Read the model definition and answer for the solid it produces. Units are mm, in the model's axes. A direction names the side the tool comes from. Coordinates: 2 decimals unless noted, no trailing zeros. Loops run counter-clockwise (first coordinate to the right, second up) from the corner with the lowest first, then second, coordinate; pieces in that order, holes last. Notation, with made-up numbers: M -30,-30 L -6,-30 A16 ccw -6,-6 Z; hole C 56,-19 d9. An arc over 180 degrees is marked long. Put each result on its own line as item: value.
from build123d import *

# Parameters (mm, degrees)
BOX_EXTRUDE_DEPTH             = 100
BOX_EXTRUDE_DEPTH_BACK        = 15
SKETCH2_W                     = 160
SKETCH2_H                     = 140
BOX_INNER_CUT_START           = -20
SKETCH3_W                     = 120
SKETCH3_H                     = 100
BOX_INNER_CUT_DEPTH           = 40
SHAFT_CUT_START               = -60
SKETCH6_R                     = 6
SHAFT_CUT_DEPTH               = 40
BEARING_CUTS_INSIDE_BOX_START = -60
SKETCH9_R                     = 8
SKETCH9_R_2                   = 16
BEARING_CUTS_INSIDE_BOX_DEPTH = 10
SKETCH11_W                    = 120
SKETCH11_H                    = 10
SCISSOR_CUT_DEPTH             = 20
SKETCH12_R                    = 16
MOTOR_HOLE_CUT_DEPTH          = 3.15
RIGHT_SHAFT_LID_CUT_REACH     = 156.306
SKETCH15_R                    = 6
LEFT_BEARING_LID_CUT_START    = -10
SKETCH18_R                    = 8
LEFT_BEARING_LID_CUT_DEPTH    = 10
OUTER_EDGES_FILLET_R          = 4


with BuildPart() as part:
    # Sketch2 → BOX_EXTRUDE (new, two sides: drawn at the far end of the back side and taken through both)
    with BuildSketch(Plane(origin=(0, 0, 0), x_dir=(1, 0, 0), z_dir=(0, 1, 0)).offset(-BOX_EXTRUDE_DEPTH_BACK)):
        Rectangle(SKETCH2_W, SKETCH2_H)
    extrude(amount=BOX_EXTRUDE_DEPTH + BOX_EXTRUDE_DEPTH_BACK)

    # Sketch3 → BOX_INNER_CUT (cut)
    with BuildSketch(Plane(origin=(0, 100, 0), x_dir=(1, 0, 0), z_dir=(0, 1, 0)).offset(BOX_INNER_CUT_START)):
        Rectangle(SKETCH3_W, SKETCH3_H)
    extrude(amount=-BOX_INNER_CUT_DEPTH, mode=Mode.SUBTRACT)

    # Sketch6 → SHAFT_CUT (cut)
    with BuildSketch(Plane(origin=(0, 100, 0), x_dir=(1, 0, 0), z_dir=(0, 1, 0)).offset(SHAFT_CUT_START)):
        with Locations(Location((15, 0, 0), (0, 0, 270))):
            Circle(SKETCH6_R)
        with Locations(Location((-15, 0, 0), (0, 0, 90))):
            Circle(SKETCH6_R)
    extrude(amount=-SHAFT_CUT_DEPTH, mode=Mode.SUBTRACT)

    # Sketch9 → BEARING_CUTS_INSIDE_BOX (cut)
    with BuildSketch(Plane(origin=(0, 100, 0), x_dir=(1, 0, 0), z_dir=(0, 1, 0)).offset(BEARING_CUTS_INSIDE_BOX_START)):
        with Locations(Location((15, 0, 0), (0, 0, 270))):
            Circle(SKETCH9_R)
        with Locations(Location((-15, 0, 0), (0, 0, 270))):
            Circle(SKETCH9_R_2)
    extrude(amount=-BEARING_CUTS_INSIDE_BOX_DEPTH, mode=Mode.SUBTRACT)

    # Sketch11 → SCISSOR_CUT (cut)
    with BuildSketch(Plane.XY.offset(70)):
        with Locations((0, 45)):
            Rectangle(SKETCH11_W, SKETCH11_H)
    extrude(amount=-SCISSOR_CUT_DEPTH, mode=Mode.SUBTRACT)

    # Sketch12 → MOTOR_HOLE_CUT (cut)
    with BuildSketch(Plane(origin=(0, 100, 0), x_dir=(1, 0, 0), z_dir=(0, 1, 0))):
        with Locations(Location((15, 0, 0), (0, 0, 270))):
            Circle(SKETCH12_R)
    extrude(amount=-MOTOR_HOLE_CUT_DEPTH, mode=Mode.SUBTRACT)

    # Sketch15 → RIGHT_SHAFT_LID_CUT (cut, up to next)
    with BuildSketch(Plane(origin=(0, 96.85, 0), x_dir=(1, 0, 0), z_dir=(0, 1, 0)), mode=Mode.PRIVATE) as right_shaft_lid_cut_sk1:
        with Locations(Location((15, 0, 0), (0, 0, 270))):
            Circle(SKETCH15_R)
    right_shaft_lid_cut_tool1 = extrude(right_shaft_lid_cut_sk1.sketch, amount=-RIGHT_SHAFT_LID_CUT_REACH, mode=Mode.PRIVATE) & part.part
    add(right_shaft_lid_cut_tool1.solids().sort_by_distance((15, 96.85, 0))[0], mode=Mode.SUBTRACT)

    # Sketch18 → LEFT_BEARING_LID_CUT (cut)
    with BuildSketch(Plane(origin=(0, 100, 0), x_dir=(1, 0, 0), z_dir=(0, 1, 0)).offset(LEFT_BEARING_LID_CUT_START)):
        with Locations(Location((-15, 0, 0), (0, 0, 270))):
            Circle(SKETCH18_R)
    extrude(amount=-LEFT_BEARING_LID_CUT_DEPTH, mode=Mode.SUBTRACT)

    # OUTER_EDGES_FILLET
    outer_edges_fillet_edges = [part.edges().sort_by_distance(p)[0] for p in [
        (-80, 42.5, -70),
        (80, 42.5, -70),
        (80, 42.5, 70),
        (-80, 42.5, 70),
    ]]
    fillet(outer_edges_fillet_edges, radius=OUTER_EDGES_FILLET_R)


solid = part.part
1) Find section A-A, the plane x = 39. Write down the section's boundary in (y, z).
Answer list:
outline: M -15,-70 L 100,-70 L 100,70 L 50,70 L 50,50 L 80,50 L 80,-50 L 40,-50 L 40,70 L -15,70 Z
2) Find section C-C, the plane x = 15. Write down the section's boundary in (y, z), plus the area to 3 significant figures.
Answer list:
outline: M -15,-70 L 100,-70 L 100,-16 L 96.85,-16 L 96.85,-6 L 80,-6 L 80,-50 L 40,-50 L 40,-8 L 30,-8 L 30,-6 L 0,-6 L 0,6 L 30,6 L 30,8 L 40,8 L 40,70 L -15,70 Z; M 50,50 L 80,50 L 80,6 L 96.85,6 L 96.85,16 L 100,16 L 100,70 L 50,70 Z
area: 11,100 mm^2
3) Which of the six approach directions +Z, -Z, +X, -X, +Y, -Y give full straight-line access (tool end or side, diameter ignored) to faces 4 (the flat face through (15, 0, 0)), 5 (the flat face through (-80, 42, 1)), 6 (the cylindrical face through (-30.62, 35.07, -3.47))?
Answer list:
face 4: +Y
face 5: +Z, -Z, -X, +Y, -Y
face 6: none
4) Straight lines are drawn through the part: line 1 (X direction, y = 14.25, z = 0); line 2 (Y direction, x = 16.5, z = 62.5); line 3 (Y direction, x = -58, z = 27.5). For each, find the intervals that lie inside material, in ascending order. Write a range as [from, to].
Answer list:
line 1: x = [-80, -21], [-9, 9], [21, 80]
line 2: y = [-15, 40], [50, 100]
line 3: y = [-15, 40], [80, 100]
5) Find section B-B, the plane y = 62. Write down the section's boundary in (x, z).
Answer list:
outline: M -80,-66 A4 ccw -76,-70 L 76,-70 A4 ccw 80,-66 L 80,66 A4 ccw 76,70 L -76,70 A4 ccw -80,66 Z; hole M -60,-50 L 60,-50 L 60,50 L -60,50 Z
6) Given pin 1 Ø5 at (x, z) = (12.5, 0) entering from +Y, flat-ended and moving along its own axis, determine where the tip first touches the part or whether it passes through.
Answer list:
pin 1: stops at y = 0
7) Determine the mould class of faces 1 (the flat face through (80, 42, 1)), 2 (the flat face through (-1, 42, -70)), 3 (the flat face through (-1, 50, 60)) for opening direction X: released by +X, released by -X, zero draft, split by the parting line, or undercut.
Answer list:
face 1: released by +X
face 2: zero draft
face 3: undercut
8) Find section D-D, the plane z = 35. Write down the section's boundary in (x, y), plus the area to 3 significant figures.
Answer list:
outline: M -80,-15 L 80,-15 L 80,100 L -80,100 Z; hole M -60,40 L 60,40 L 60,80 L -60,80 Z
area: 13,600 mm^2
